Check sheet for the modelled part. Datum: model origin and axes. Units: mm. Face numbers are marked on the shaded views. Round coordinates to 2 decimals unless told otherwise and drop trailing zeros. Write each loop counter-clockwise with the first axis right and the second up, starting at its lowest first coordinate (ties: lowest second). Pieces come first, ordered by that corner, then holes. Notation, with made-up numbers: (33, -31) -> (53, -31) arc R7 cw to (53, -20) -> close; hole circle Ø7 at (-1.75, -18). An arc over 180 degrees is marked (long way). One line per item, written item: value.
from build123d import *

# Parameters (mm, degrees)
F0_W     = 127
F0_H     = 127
F1_DEPTH = 45.974
F2_R     = 2.54
F3_T     = 2.54


# Not quite as in the source:
# - a shell that OpenCascade refuses in one call is made with other operations: the cavity is built on its own and cut out


with BuildPart() as f1:
    # F0 (on Front) → F1 (new body, symmetric)
    with BuildSketch(Plane.XZ):
        with Locations((-0.4519568912, 63.5)):
            Rectangle(F0_W, F0_H)
    extrude(amount=F1_DEPTH, both=True)

    # F2
    f2_edges = [f1.edges().sort_by_distance(p)[0] for p in [
        (-63.951957, -45.974, 63.5),
        (63.048043, -45.974, 63.5),
        (63.048043, 45.974, 63.5),
        (-63.951957, 45.974, 63.5),
    ]]
    fillet(f2_edges, radius=F2_R)

    # F3: shell of thickness 2.54, made by hand


with BuildPart() as f3_core1:
    # F3_t2: copy of F1
    add(f1.part)

    # the walls: a layer under each face that stays
    f3_faces = [f3_core1.faces().sort_by_distance(p)[0] for p in [
        (-0.4519568912, 45.974, 63.5),
        (63.0480431088, 0, 63.5),
        (-63.9519568912, 0, 63.5),
        (-0.4519568912, -45.974, 63.5),
        (-0.4519568912, 0, 0),
    ]]
    thicken(f3_faces, amount=-F3_T, mode=Mode.SUBTRACT)


with BuildPart() as f1_1:
    add(f1.part)

    # what is left inside the walls is the cavity
    f3_cavity = [f3_core1.part.solids().sort_by_distance(p)[0] for p in [
        (-0.451957, -43.4086, 44.026667),
    ]]
    add(f3_cavity, mode=Mode.SUBTRACT)


solid = f1_1.part
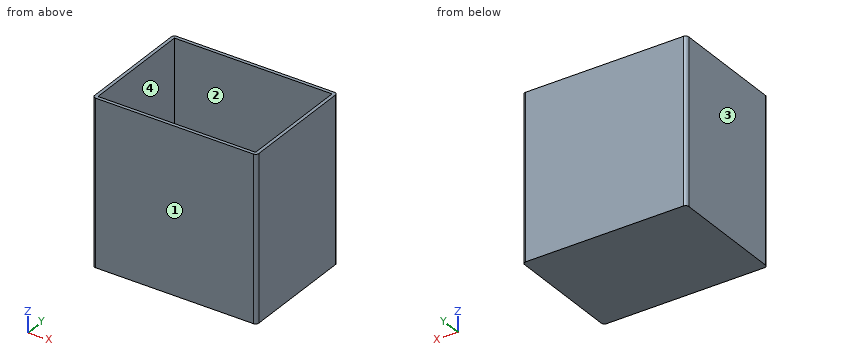
Item 1: Depth check by flat-ended pin: pin 1 (12 mm diameter, centred on x = -27.5, y = 20.5, fed in from +Z). Enter the tip coordinate at first touch or a pass-through.
Result set:
pin 1: z = 2.54
Item 2: Sectioned sample at B-B (z = 113). Enter the section's corners in (x, y).
Result set:
outline: (-63.95, -43.43) arc R2.54 ccw to (-61.41, -45.97) -> (60.51, -45.97) arc R2.54 ccw to (63.05, -43.43) -> (63.05, 43.43) arc R2.54 ccw to (60.51, 45.97) -> (-61.41, 45.97) arc R2.54 ccw to (-63.95, 43.43) -> close; hole (-61.41, -43.43) -> (60.51, -43.43) -> (60.51, 43.43) -> (-61.41, 43.43) -> close
Item 3: Material ranges on line 1 along Y through (x, z) = (-53, 83); line 2 along X through (y, z) = (-38, 70); line 3 along Z through (x, y) = (34.5, -23.5), recorded low to high.
Result set:
line 1: -45.97 to -43.43, 43.43 to 45.97
line 2: -63.95 to -61.41, 60.51 to 63.05
line 3: 0 to 2.54
Item 4: Release check for a two-part mould opening along X. For the marked faces 1, 2, 3 and 4 record: pulls with the +X half, pulls with the -X half, needs draft (parallel to the pull), parting line crosses it, or undercut.
Result set:
face 1: needs draft
face 2: undercut
face 3: pulls with the -X half
face 4: undercut
Item 5: Sectioned sample at C-C (x = 41). Enter the section's corners in (y, z), then the cut area to 3 significant figures.
Result set:
outline: (-45.97, 0) -> (45.97, 0) -> (45.97, 127) -> (43.43, 127) -> (43.43, 2.54) -> (-43.43, 2.54) -> (-43.43, 127) -> (-45.97, 127) -> close
area: 866 mm^2
Item 6: Sectioned sample at A-A (y = 11). Enter the section's corners in (x, z), then the cut area to 3 significant figures.
Result set:
outline: (-63.95, 0) -> (63.05, 0) -> (63.05, 127) -> (60.51, 127) -> (60.51, 2.54) -> (-61.41, 2.54) -> (-61.41, 127) -> (-63.95, 127) -> close
area: 955 mm^2
